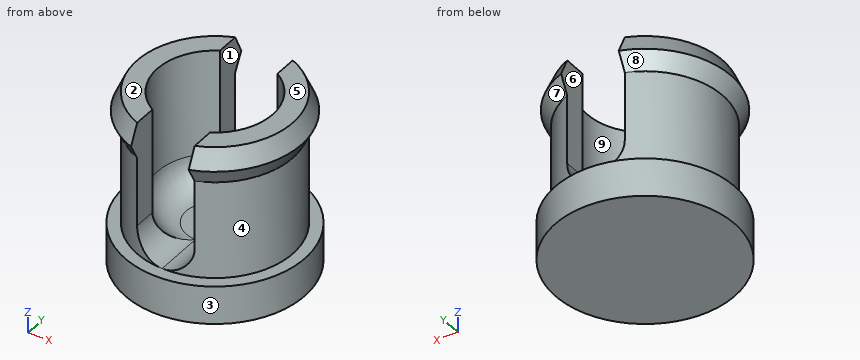
from build123d import *

# Parameters (mm, degrees)
F3_R     = 7.62
F4_DEPTH = 17.78
F6_DEPTH = 25.4
F7_R     = 3.80999


# Not quite as in the source:
# - a fillet or chamfer is up to 0.001 mm smaller than in the source, because OpenCascade refuses the exact size


with BuildPart() as f2:
    # F0 (on Front) → F2 (revolve)
    with BuildSketch(Plane.XZ):
        Polygon((-11.90625, 5.08), (-11.90625, 0), (0, 0), (0, 22.86), (-10.31875, 22.86), (-11.43, 20.32), (-10.31875, 18.0785163727), (-10.31875, 5.08), align=None)
    revolve(axis=Axis((0, 0, 7.382690208), (0, 0, 1)))

    # F3 (on face) → F4 (cut, through all)
    with BuildSketch(Plane.XY.offset(22.86)):
        Circle(F3_R)
    extrude(amount=-F4_DEPTH, mode=Mode.SUBTRACT)

    # F5 (on face) → F6 (cut)
    with BuildSketch(Plane.XY.offset(5.08)):
        Polygon((3.81, 14.0309315175), (-3.81, 14.0309315175), (-3.81, 3.81), (-3.81, -15.0898629799), (3.81, -15.0898629799), (3.81, 3.81), align=None)
    extrude(amount=F6_DEPTH, mode=Mode.SUBTRACT)

    # F7 (radius 3.81 in the source; OpenCascade refuses exactly that, so slightly less here)
    f7_edges = [f2.edges().sort_by_distance(p)[0] for p in [
        (-7.62, 0, 5.08),
        (7.62, 0, 5.08),
        (3.81, 8.094359, 5.08),
        (3.81, -8.094359, 5.08),
        (-3.81, -8.094359, 5.08),
        (-3.81, 8.094359, 5.08),
    ]]
    fillet(f7_edges, radius=F7_R)


solid = f2.part
For this review, take the finished solid that the model builds, in its own axes (mm). Face numbers are marked on the shaded views. A direction names the side the tool comes from. Give positions to 0.01 mm unless a question says otherwise; leave off trailing zeros. Loops run counter-clockwise (first coordinate to the right, second up) from the corner with the lowest first, then second, coordinate; pieces in that order, holes last. Notation, with made-up numbers: M -15,72.25 L 43,72.25 A24 ccw 43,110.25 Z; hole C 53.5,3.25 d9. An arc over 180 degrees is marked long. Answer as a JSON object with one key per item and string values. Group by question number.
Q1. Mouldability with a two-part tool opening along X and no side actions: class the marked faces 1, 2, 3 and 4 as +X half, -X half, draft (parallel to the pull), parting line (faces both ways), or undercut.
Q2. Add section A-A on z = 12. Give the boundary of the cut face in (x, y).
Q3. Add section B-B on y = 0. Give the boundary of the cut face in (x, z).
Q4. Tool access review of the marked faces 5, 6, 7, 8 and 9: name each direction out of +Z, -Z, +X, -X, +Y, -Y from which nothing blocks a thin tool from reaching the whole face with its end or side.
Q5. Add section C-C on z = 2. Give the boundary of the cut face in (x, y), and give its area (3 significant figures).
Q6. Insertion check: P1, Ø3.5, axis at y = 8.5, z = 12.5, coming from the +X side; P2, Ø4, axis at x = -6, z = 17, coming from the +Y side; P3, Ø2, axis at x = 8, z = 12, coming from the -Y side; P4, Ø3, axis at x = 0.5, z = 15, coming from the +Y side. Each pin has a flat end and moves straight along its axis. Give the tip position at first contact, or say it passes through.
Q7. For probe 1 along Z at (x, y) = (1.5, -11); probe 2 along X at (y, z) = (-2.5, 6); probe 3 along Y at (x, z) = (5.25, 16.5), list the stretches that pass through material, from the lowest coordinate up. Write a range as [from, to].
Checked values:
{
 "1": {"face 1": "undercut", "face 2": "draft", "face 3": "parting line", "face 4": "+X half"},
 "2": {"outline": "M -3.81,-9.59 L -3.81,-6.6 A7.62 cw -3.81,6.6 L -3.81,9.59 A10.32 ccw Z; M 3.81,-9.59 A10.32 ccw 3.81,9.59 L 3.81,6.6 A7.62 cw 3.81,-6.6 Z"},
 "3": {"outline": "M -11.91,0 L 11.91,0 L 11.91,5.08 L 10.32,5.08 L 10.32,18.08 L 11.43,20.32 L 10.32,22.86 L 7.62,22.86 L 7.62,8.89 A3.81 cw 3.81,5.08 L -3.81,5.08 A3.81 cw -7.62,8.89 L -7.62,22.86 L -10.32,22.86 L -11.43,20.32 L -10.32,18.08 L -10.32,5.08 L -11.91,5.08 Z"},
 "4": {"face 5": "+Z, +X, -X, +Y, -Y", "face 6": "+Z, +Y, -Y", "face 7": "+X", "face 8": "-X", "face 9": "+Z"},
 "5": {"outline": "C 0,0 d23.81", "area": "445 mm²"},
 "6": {"P1": "x = 7.8", "P2": "y = 9.51", "P3": "y = -7.58", "P4": "through"},
 "7": {"probe 1": "[0, 5.08]", "probe 2": "[-10.01, -5.77], [5.77, 10.01]", "probe 3": "[-8.88, -5.52], [5.52, 8.88]"}
}
